```python
from build123d import *

# Parameters (mm, degrees)
SALIENTE_EXTRUIR1_DEPTH = 43.8
CHAFL_N1_SIZE           = 20
CROQUIS2_R              = 30
CROQUIS2_R_2            = 20
SALIENTE_EXTRUIR2_DEPTH = 13.5
REDONDEO1_R             = 2


with BuildPart() as part:
    # Croquis1 → Saliente-Extruir1 (new body)
    with BuildSketch(Plane(origin=(0, 0, 0), x_dir=(1, 0, 0), z_dir=(0, 1, 0))):
        with BuildLine():
            Line((-10, -58.530413525), (-10, -80))
            Line((-10, -80), (10, -80))
            Line((10, -80), (10, -58.530413525))
            ThreePointArc((10, -58.530413525), (41.986958138, -41.986958138), (58.530413525, -10))
            Line((58.530413525, -10), (80, -10))
            Line((80, -10), (80, 10))
            Line((80, 10), (58.530413525, 10))
            ThreePointArc((58.530413525, 10), (41.986958138, 41.986958138), (10, 58.530413525))
            Line((10, 58.530413525), (10, 80))
            Line((10, 80), (-10, 80))
            Line((-10, 80), (-10, 58.530413525))
            ThreePointArc((-10, 58.530413525), (-41.986958138, 41.986958138), (-58.530413525, 10))
            Line((-58.530413525, 10), (-80, 10))
            Line((-80, 10), (-80, -10))
            Line((-80, -10), (-58.530413525, -10))
            ThreePointArc((-58.530413525, -10), (-41.986958138, -41.986958138), (-10, -58.530413525))
        make_face()
    extrude(amount=SALIENTE_EXTRUIR1_DEPTH)

    # Chaflán1
    chafl_n1_edges = [part.edges().sort_by_distance(p)[0] for p in [
        (-80, 43.8, 0),
        (-41.986958138, 43.8, 41.986958138),
        (0, 43.8, 80),
        (41.986958138, 43.8, 41.986958138),
        (80, 43.8, 0),
        (41.986958138, 43.8, -41.986958138),
        (0, 43.8, -80),
        (-41.986958138, 43.8, -41.986958138),
    ]]
    chamfer(chafl_n1_edges, length=CHAFL_N1_SIZE)

    # Croquis2 → Saliente-Extruir2 (add)
    with BuildSketch(Plane(origin=(0, 43.8, 0), x_dir=(1, 0, 0), z_dir=(0, 1, 0))):
        Circle(CROQUIS2_R)
        Circle(CROQUIS2_R_2, mode=Mode.SUBTRACT)
    extrude(amount=SALIENTE_EXTRUIR2_DEPTH)

    # Redondeo1
    redondeo1_edges = [part.edges().sort_by_distance(p)[0] for p in [
        (-20, 43.8, 0),
        (-30, 57.3, 0),
        (-20, 57.3, 0),
    ]]
    fillet(redondeo1_edges, radius=REDONDEO1_R)


solid = part.part
```
Input: part model. Units: mm. Frame: model coordinates. A direction names the side the tool comes from. Give positions to 0.01 mm unless a question says otherwise; leave off trailing zeros. Write each loop counter-clockwise with the first axis right and the second up, starting at its lowest first coordinate (ties: lowest second). Pieces come first, ordered by that corner, then holes. Notation, with made-up numbers: (38, -22.5) - (95, -22.5) arc R31 cw to (95, 12.5) - close; hole circle Ø3 at (46, 87). An arc over 180 degrees is marked (long way). Write item = value, one per line. Start each with the question number.
1. Section query B-B, the plane z = 0. Output: boundary loops of the cut face in (x, y).
2. Access query for faces 4 (the flat face through (-14, 43.8, -27)), 5 (the flat face through (-10, 22, -64)), 6 (the flat face through (-10, 22, 63)). Directions: +Z, -Z, +X, -X, +Y, -Y. A direction counts if a zero-diameter tool reaches every point of the face in a straight line with its end or side. Return the directions, or none.
3. Ray query, L1, parallel to Z at x = 0, y = 52; L2, parallel to Y at x = -8, z = -31. Return the intervals inside material, ascending.
4. Section query A-A, the plane y = 50. Output: boundary loops of the cut face in (x, z).
5. Section query C-C, the plane x = 0. Output: boundary loops of the cut face in (y, z).
6. Mould query, pull axis X, two halves, no side actions, for faces 1 (the flat face through (64, 22, -10)), 2 (the cylindrical face through (-41.62, 11.73, -42.35)), 3 (the cylindrical face through (-4.336, 50.484, 19.524)). Classes: released by +X, released by -X, zero draft, split by the parting line, or undercut.
7. First-contact query: pin 1 Ø12.5 at (y, z) = (23.5, 50.5) entering from +X; pin 2 Ø1.5 at (x, z) = (28.5, -48) entering from -Y; pin 3 Ø21 at (x, y) = (-49.5, 26) entering from +Z; pin 4 Ø12.5 at (x, y) = (67.5, 15.5) entering from +Z. Flat tips, straight axial feed; report the tip coordinate or a pass-through.
8. Section query D-D, the plane y = 26. Output: boundary loops of the cut face in (x, z).
Check sheet entries:
q1.outline = (-80, 0) - (80, 0) - (80, 23.8) - (60, 43.8) - (30, 43.8) - (30, 55.3) arc R2 ccw to (28, 57.3) - (22, 57.3) arc R2 ccw to (20, 55.3) - (20, 45.8) arc R2 cw to (18, 43.8) - (-18, 43.8) arc R2 cw to (-20, 45.8) - (-20, 55.3) arc R2 ccw to (-22, 57.3) - (-28, 57.3) arc R2 ccw to (-30, 55.3) - (-30, 43.8) - (-60, 43.8) - (-80, 23.8) - close
q2.face_4 = +Y
q2.face_5 = -Z, -X, +Y
q2.face_6 = +Z, -X, +Y
q3.L1 = -30 to -20, 20 to 30
q3.L2 = 0 to 43.8
q4.outline = circle Ø60 at (0, 0); hole circle Ø40 at (0, 0)
q5.outline = (0, -80) - (23.8, -80) - (43.8, -60) - (43.8, -30) - (55.3, -30) arc R2 ccw to (57.3, -28) - (57.3, -22) arc R2 ccw to (55.3, -20) - (45.8, -20) arc R2 cw to (43.8, -18) - (43.8, 18) arc R2 cw to (45.8, 20) - (55.3, 20) arc R2 ccw to (57.3, 22) - (57.3, 28) arc R2 ccw to (55.3, 30) - (43.8, 30) - (43.8, 60) - (23.8, 80) - (0, 80) - close
q6.face_1 = zero draft
q6.face_2 = released by -X
q6.face_3 = undercut
q7.pin_1 = 39.59
q7.pin_2 = 0
q7.pin_3 = 44.57
q7.pin_4 = 10
q8.outline = (-77.8, -10) - (-56.3, -10) arc R57.18 ccw to (-10, -56.3) - (-10, -77.8) - (10, -77.8) - (10, -56.3) arc R57.18 ccw to (56.3, -10) - (77.8, -10) - (77.8, 10) - (56.3, 10) arc R57.18 ccw to (10, 56.3) - (10, 77.8) - (-10, 77.8) - (-10, 56.3) arc R57.18 ccw to (-56.3, 10) - (-77.8, 10) - close
